Could you check a few things on this model? Use its own coordinates, in mm. Face numbers are marked on the shaded views. A direction names the side the tool comes from. Coordinates: 2 decimals unless noted, no trailing zeros. Loops run counter-clockwise (first coordinate to the right, second up) from the corner with the lowest first, then second, coordinate; pieces in that order, holes last.
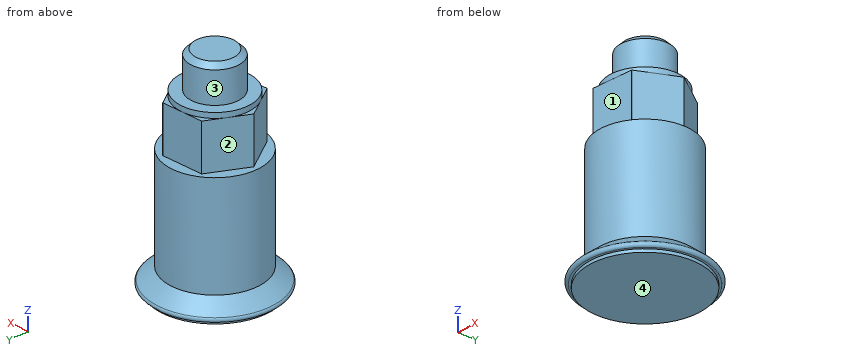
from build123d import *

# Parameters (mm, degrees)
SKETCH_1_R               = 4.5
EXTRUDE_1_DEPTH          = 10
SKETCH_1_2_R             = 4.5
EXTRUDE_2_DEPTH          = 1.6
EXTRUDE_2_DRAFT          = 50
FILLET_1_R               = 0.25
SKETCH_5_R               = 5.5
EXTRUDE_3_DEPTH          = 0.3
EXTRUDE_4_DEPTH          = 4.5
PATTERN_CIRCULAR_1_COUNT = 6
SKETCH_8_R               = 3.5
EXTRUDE_5_DEPTH          = 0.5
SKETCH_9_R               = 2.413
EXTRUDE_6_DEPTH          = 3.5
CHAMFER_1_SIZE           = 0.48


with BuildPart() as part:
    # Sketch 1 → Extrude 1 (new body)
    with BuildSketch(Plane.XY):
        Circle(SKETCH_1_R)
    extrude(amount=EXTRUDE_1_DEPTH)


with BuildPart() as extrude_2_tool:
    # Sketch 1_2 → Extrude 2 (with draft: the straight prism first)
    with BuildSketch(Plane.XY):
        Circle(SKETCH_1_2_R)
    extrude(amount=-EXTRUDE_2_DEPTH)
    # Extrude 2: the draft: its side faces are tilted about the plane it starts from
    extrude_2_sides = [extrude_2_tool.faces().sort_by_distance(p)[0] for p in [
        (-4.5, 0, -0.8),
    ]]
    draft(extrude_2_sides, Plane.XY, EXTRUDE_2_DRAFT)


with BuildPart() as part_1:
    add(part.part)

    # Extrude 2: add extrude_2_tool
    add(extrude_2_tool.part)

    # Fillet 1
    fillet_1_edges = [part_1.edges().sort_by_distance(p)[0] for p in [
        (-6.406805748, 0, -1.6),
    ]]
    fillet(fillet_1_edges, radius=FILLET_1_R)

    # Sketch 5 → Extrude 3 (add)
    with BuildSketch(Plane(origin=(0, 0, -1.6), x_dir=(-1, 0, 0), z_dir=(0, 0, -1))):
        with Locations(Location((0, 0, 0), (0, 0, 180))):
            Circle(SKETCH_5_R)
    extrude(amount=EXTRUDE_3_DEPTH)

    # Sketch 7 → Extrude 4 (add)
    with BuildSketch(Plane.XY.offset(10)):
        Polygon((0, 0), (-2.201088416, 3.388936527), (1.839911584, 3.597833565), align=None)
    extrude_4 = extrude(amount=EXTRUDE_4_DEPTH)

    # Pattern Circular 1: Extrude 4 ×6 about axis
    pattern_circular_1_axis = Axis((0, 0, 0), (0, 0, 1))
    for i in range(1, PATTERN_CIRCULAR_1_COUNT):
        add(extrude_4.rotate(pattern_circular_1_axis, i * 360 / PATTERN_CIRCULAR_1_COUNT))

    # Sketch 8 → Extrude 5 (add)
    with BuildSketch(Plane.XY.offset(14.5)):
        with Locations(Location((0, 0, 0), (0, 0, 154.872089373))):
            Circle(SKETCH_8_R)
    extrude(amount=EXTRUDE_5_DEPTH)

    # Sketch 9 → Extrude 6 (add)
    with BuildSketch(Plane.XY.offset(15)):
        Circle(SKETCH_9_R)
    extrude(amount=EXTRUDE_6_DEPTH)

    # Chamfer 1
    chamfer_1_edges = [part_1.edges().sort_by_distance(p)[0] for p in [
        (-2.413, 0, 18.5),
    ]]
    chamfer(chamfer_1_edges, length=CHAMFER_1_SIZE)


solid = part_1.part
(1) I need wall thicknesses on probe 1 along Z at (x, y) = (1.5, -2); probe 2 along Z at (x, y) = (0, 4); probe 3 along X at (y, z) = (-2, 3.5). Which ranges of each line are inside material? Lowest first, please.
Answers:
probe 1: z = -1.9 to 15
probe 2: z = -1.9 to 10
probe 3: x = -4.03 to 4.03
(2) Imagine slicing it at B-B, the plane z = 7.75. Write out the boundary of the cut face in (x, y), and give its area (3 significant figures).
Answers:
outline: circle Ø9 at (0, 0)
area: 63.6 mm2
(3) Which directions (+Z, -Z, +X, -X, +Y, -Y) give clear straight access to the entire face, cutting with the end or side of a thin tool? Please do the marked faces 1, 2, 3 and 4.
Answers:
face 1: +Z, +X, -Y
face 2: +Z, -X, +Y
face 3: +Z
face 4: -Z, +X, -X, +Y, -Y
(4) For pin 1 (1.3 mm diameter, centred on x = 0.5, y = 2.5, fed in from +Z); pin 2 (4 mm diameter, centred on y = 0, z = 16, fed in from +X); pin 3 (1.1 mm diameter, centred on x = 3.5, y = 0, fed in from +Z); pin 4 (1 mm diameter, centred on x = 4, z = 3, fed in from -Y), each with a flat end and sliding along its axis, tell me the tip position at first contact or that it passes through.
Answers:
pin 1: stops at z = 18.5
pin 2: stops at x = 4.04
pin 3: stops at z = 15
pin 4: stops at y = -2.83
